```python
from build123d import *

# Parameters (mm, degrees)
BOSS_EXTRUDE1_DEPTH = 220
BOSS_EXTRUDE2_DEPTH = 3
FILLET1_R           = 1.5
SCALE1_SCALE        = 15.6
SCALE2_SCALE        = 0.5


with BuildPart() as part:
    # Sketch1 → Boss-Extrude1 (new body)
    with BuildSketch(Plane.XY):
        with BuildLine():
            Line((0, 0), (0, -4.480629882))
            Line((0, -4.480629882), (6.620887994, -4.480629882))
            ThreePointArc((6.620887994, -4.480629882), (11.673872347, -6.882935474), (16.9859081, -8.639636697))
            Line((16.9859081, -8.639636697), (16.9859081, -13.120266579))
            ThreePointArc((16.9859081, -13.120266579), (28.43159427, -14.466004542), (39.877280439, -13.120266579))
            Line((39.877280439, -13.120266579), (39.877280439, -8.639636697))
            ThreePointArc((39.877280439, -8.639636697), (45.189316192, -6.882935474), (50.242300545, -4.480629882))
            Line((50.242300545, -4.480629882), (56.863188539, -4.480629882))
            Line((56.863188539, -4.480629882), (56.863188539, 0))
            Line((56.863188539, 0), (0, 0))
        make_face()
    extrude(amount=BOSS_EXTRUDE1_DEPTH)

    # Sketch2 → Boss-Extrude2 (add)
    with BuildSketch(Plane.XY.offset(220)):
        Polygon((6.620887994, 0), (12.113374984, 6.832485321), (44.749813555, 6.832485321), (50.242300545, 0), (48.317723739, 0), (44.031054266, 5.332485321), (12.832134273, 5.332485321), (8.545464801, 0), align=None)
    extrude(amount=-BOSS_EXTRUDE2_DEPTH)

    # Fillet1
    fillet1_edges = [part.edges().sort_by_distance(p)[0] for p in [
        (12.113374984, 6.832485321, 218.5),
        (44.749813555, 6.832485321, 218.5),
    ]]
    fillet(fillet1_edges, radius=FILLET1_R)


with BuildPart() as part_1:
    # Scale1: scaled about (28.43159427, -5.503767505, 110.201488626)
    add(part.part.scale(SCALE1_SCALE).moved(Location((-415.101276342, 80.355005573, -1608.94173394))))


with BuildPart() as part_2:
    # Scale2: scaled about (28.431594264, -5.503767501, 110.201488629)
    add(part_1.part.scale(SCALE2_SCALE).moved(Location((14.215797132, -2.75188375, 55.100744314))))


solid = part_2.part
```
CAD build for the part. Positions are in the model's coordinates, mm. A direction names the side the tool comes from. Coordinates: 2 decimals unless noted, no trailing zeros. Order: outer loops, then holes, each group sorted by start corner. A loop starts at its lowest first (then second) coordinate and runs counter-clockwise, first axis right, second up. Notation, with made-up numbers: (89.5, 32.25) - (127.5, 32.25) arc R26 ccw to (127.5, 51.25) - close; hole circle Ø7 at (-14, 43). An arc over 180 degrees is marked (long way). Answer in a Markdown table with one row per item.
1. Drill centre lines: L1, parallel to Y at x = -149, z = -199; L2, parallel to Y at x = 23, z = 696; L3, parallel to Z at x = -129, y = 51.5. Where is each one in solid material? Low to high. Write a range as from..to.
Answer:
| item | result |
|---|---|
| L1 | 2.48..37.43 |
| L2 | -75.37..37.43 |
| L3 | 943.23..966.63 |
2. Flat gauge pins, fed straight in: P1, Ø2, axis at x = -143.5, z = -434, coming from the -Y side; P2, Ø4, axis at x = -100, z = 632.5, coming from the -Y side; P3, Ø5, axis at x = -134.5, z = 540, coming from the +Y side. Where does each tip first touch, or does it go through?
Answer:
| item | result |
|---|---|
| P1 | y = 2.48 |
| P2 | y = -17.95 |
| P3 | y = 37.43 |
3. Slice it at A-A, the plane z = -55. List the corners of the cut face in (x, y), then the cut area to 3 significant figures.
Answer:
| item | result |
|---|---|
| outline | (-193.33, 2.48) - (-141.69, 2.48) arc R351 ccw to (-60.84, -29.96) - (-60.84, -64.91) arc R384.9 ccw to (117.71, -64.91) - (117.71, -29.96) arc R351 ccw to (198.56, 2.48) - (250.2, 2.48) - (250.2, 37.43) - (-193.33, 37.43) - close |
| area | 31,700 mm² |
4. Slice it at B-B, the plane y = 55.5. List the corners of the cut face in (x, z), then the cut area to 3 significant figures.
Answer:
| item | result |
|---|---|
| outline | (-127.16, 943.23) - (-112.15, 943.23) - (-112.15, 966.63) - (-127.16, 966.63) - close; (169.01, 943.23) - (184.03, 943.23) - (184.03, 966.63) - (169.01, 966.63) - close |
| area | 703 mm² |
5. Pull direction X, two halves, no side cores. Call faces 5 (the face through (-193.335, 20, 97)), 6 (the face through (158.57, -16.49, 96.62)), 7 (the face through (-109.73, 58.51, 955.09)), 8 (the face through (25, -6, -749.37)): +X half, -X half, draft (parallel to the pull), parting line (faces both ways), or undercut.
Answer:
| item | result |
|---|---|
| face 5 | -X half |
| face 6 | +X half |
| face 7 | undercut |
| face 8 | draft |
6. 3-axis set-ups, long thin cutter, end or side, ignore diameter. For faces 1 (the face through (-60.845, -47, 97)), 2 (the face through (-122.3, 61.55, 955.09)), 3 (the face through (29, 80, 943.23)), 4 (the face through (224, 2.477, 97)): which of +Z, -Z, +X, -X, +Y, -Y reach the whole face in a straight line?
Answer:
| item | result |
|---|---|
| face 1 | +Z, -Z, -X, -Y |
| face 2 | +Z, -Z, -X, +Y |
| face 3 | -Z, +X, -X, +Y |
| face 4 | +Z, -Z, +X, -Y |
